```python
from build123d import *

# Parameters (mm, degrees)
CYLINDER008_R           = 7.1
CYLINDER008_DEPTH       = 10
BOX005_W                = 21
BOX005_H                = 17
BOX005_DEPTH            = 8
CYLINDER005_R           = 2.5
CYLINDER005_DEPTH       = 10
CYLINDER004_R           = 0.25
CYLINDER004_DEPTH       = 10
CYLINDER004_PITCH_ANGLE = 90
CYLINDER003_R           = 0.25
CYLINDER003_DEPTH       = 10
CYLINDER003_PITCH_ANGLE = 90
BOX002_W                = 6.5
BOX002_H                = 4.8
BOX002_DEPTH            = 1
BOX003_W                = 10
BOX003_H                = 12
BOX003_DEPTH            = 3
BOX001_W                = 14
BOX001_H                = 10
BOX001_DEPTH            = 7.25


with BuildPart() as cylinder008:
    # Cylinder008 → Cylinder008 (new body)
    with BuildSketch(Plane.XY.offset(-6.5)):
        Circle(CYLINDER008_R)
    extrude(amount=CYLINDER008_DEPTH)


with BuildPart() as cube005:
    # Box005 → Box005 (new body)
    with BuildSketch(Plane(origin=(-9, -7, -3.5), x_dir=(1, 0, 0), z_dir=(0, 0, 1))):
        with Locations((10.5, 8.5)):
            Rectangle(BOX005_W, BOX005_H)
    extrude(amount=BOX005_DEPTH)


with BuildPart() as cylinder005:
    # Cylinder005 → Cylinder005 (new body)
    with BuildSketch(Plane.XY.offset(0.5)):
        Circle(CYLINDER005_R)
    extrude(amount=CYLINDER005_DEPTH)


with BuildPart() as fusion004:
    # Sphere001 → Sphere001 (revolve)
    with BuildSketch(Plane.XZ):
        with BuildLine():
            ThreePointArc((0, -3.1), (3.1, 0), (0, 3.1))
            Line((0, 3.1), (0, -3.1))
        make_face()
    revolve(axis=Axis((0, 0, 0), (0, 0, 1)))

    # Fusion004: union Cylinder005
    add(cylinder005.part)


with BuildPart() as cylinder004:
    # Cylinder004 → Cylinder004 (new body)
    with BuildSketch(Plane.XY):
        Circle(CYLINDER004_R)
    extrude(amount=CYLINDER004_DEPTH)


with BuildPart() as cylinder004_1:
    # Cylinder004 pitch: moved
    add(cylinder004.part.rotate(Axis((0, 0, 0), (0, 1, 0)), CYLINDER004_PITCH_ANGLE))


with BuildPart() as cylinder004_2:
    # Cylinder004 placement: moved
    add(cylinder004_1.part.moved(Location((0, -2, -3.7))))


with BuildPart() as fusion:
    # Cylinder003 → Cylinder003 (new body)
    with BuildSketch(Plane.XY):
        Circle(CYLINDER003_R)
    extrude(amount=CYLINDER003_DEPTH)


with BuildPart() as fusion_1:
    # Cylinder003 pitch: moved
    add(fusion.part.rotate(Axis((0, 0, 0), (0, 1, 0)), CYLINDER003_PITCH_ANGLE))


with BuildPart() as fusion_2:
    # Cylinder003 placement: moved
    add(fusion_1.part.moved(Location((-11, 2, -3.7))))

    # Fusion: union Cylinder004
    add(cylinder004_2.part)


with BuildPart() as fusion001:
    # Box002 → Box002 (new body)
    with BuildSketch(Plane(origin=(-3.25, -2.4, -4.2), x_dir=(1, 0, 0), z_dir=(0, 0, 1))):
        with Locations((3.25, 2.4)):
            Rectangle(BOX002_W, BOX002_H)
    extrude(amount=BOX002_DEPTH)

    # Fusion001: union Fusion
    add(fusion_2.part)


with BuildPart() as cube003:
    # Box003 → Box003 (new body)
    with BuildSketch(Plane(origin=(-5, -6, -3.5), x_dir=(1, 0, 0), z_dir=(0, 0, 1))):
        with Locations((5, 6)):
            Rectangle(BOX003_W, BOX003_H)
    extrude(amount=BOX003_DEPTH)


with BuildPart() as switch_plate:
    # Box001 → Box001 (new body)
    with BuildSketch(Plane(origin=(-7, -5, -6), x_dir=(1, 0, 0), z_dir=(0, 0, 1))):
        with Locations((7, 5)):
            Rectangle(BOX001_W, BOX001_H)
    extrude(amount=BOX001_DEPTH)

    # Cut: cut Cube003
    add(cube003.part, mode=Mode.SUBTRACT)

    # Cut001: cut Fusion001
    add(fusion001.part, mode=Mode.SUBTRACT)

    # Cut003: cut Fusion004
    add(fusion004.part, mode=Mode.SUBTRACT)

    # Cut004: cut Cube005
    add(cube005.part, mode=Mode.SUBTRACT)

    # Common002: intersect Cylinder008
    add(cylinder008.part, mode=Mode.INTERSECT)


solid = switch_plate.part
```
CAD build for the part. Positions are in the model's coordinates, mm. Coordinates: 2 decimals unless noted, no trailing zeros. Order: outer loops, then holes, each group sorted by start corner. A loop starts at its lowest first (then second) coordinate and runs counter-clockwise, first axis right, second up.
(1) Saw through at D-D, the plane x = -5.5. Write the cut outline in (y, z), and give its area (3 significant figures).
Solution:
outline: (-4.49, -6) - (4.49, -6) - (4.49, -3.5) - (2.15, -3.5) arc R0.25 cw (long way) to (1.85, -3.5) - (-4.49, -3.5) - close
area: 22.3 mm2
(2) Mould opens along X. For faces 1 (the face through (-6.33, -3.22, -4.77)), 2 (the face through (0, 5, -5)), 3 (the face through (7, 0, -5)), 4 (the face through (0, 0, -4.2)) say: released by +X, released by -X, zero draft, split by the parting line, or undercut.
Solution:
face 1: released by -X
face 2: zero draft
face 3: released by +X
face 4: undercut
(3) Saw through at C-C, the plane z = -3.7. Write the cut outline in (x, y), and give its area (3 significant figures).
Solution:
outline: (-7, -1.19) arc R7.1 ccw to (-5.04, -5) - (5.04, -5) arc R7.1 ccw to (6.73, -2.25) - (3.25, -2.25) - (3.25, -2.4) - (-3.25, -2.4) - (-3.25, 1.75) - (-6.88, 1.75) arc R7.1 ccw to (-7, 1.19) - close; (-6.73, 2.25) - (-3.25, 2.25) - (-3.25, 2.4) - (3.25, 2.4) - (3.25, -1.75) - (6.88, -1.75) arc R7.1 ccw to (7, -1.19) - (7, 1.19) arc R7.1 ccw to (5.04, 5) - (-5.04, 5) arc R7.1 ccw to start
area: 94.1 mm2
(4) Drill centre lines: L1, parallel to Z at x = -5.15, y = 2; L2, parallel to Y at x = -4.6, z = -3.7; L3, parallel to X at y = 2.25, z = -3.9. Where is each one in solid material? Low to high.
Solution:
L1: z = -6 to -3.95
L2: y = -5 to 1.75, 2.25 to 5
L3: x = -6.73 to -3.25, 3.25 to 6.73
(5) Saw through at B-B, the plane z = -4.45. Write the cut outline in (x, y).
Solution:
outline: (-7, -1.19) arc R7.1 ccw to (-5.04, -5) - (5.04, -5) arc R7.1 ccw to (7, -1.19) - (7, 1.19) arc R7.1 ccw to (5.04, 5) - (-5.04, 5) arc R7.1 ccw to (-7, 1.19) - close
(6) Saw through at A-A, the plane y = 0. Write the cut outline in (x, z), and give its area (4 significant figures).
Solution:
outline: (-7, -6) - (7, -6) - (7, -3.5) - (3.25, -3.5) - (3.25, -4.2) - (-3.25, -4.2) - (-3.25, -3.5) - (-7, -3.5) - close
area: 30.45 mm2
